Geometry check sheet. Reference: the model listing, model coordinates, mm. A direction names the side the tool comes from. Coordinates: 2 decimals unless noted, no trailing zeros. Loops run counter-clockwise (first coordinate to the right, second up) from the corner with the lowest first, then second, coordinate; pieces in that order, holes last.
from build123d import *

# Parameters (mm, degrees)
SKETCH1_W                     = 154
SKETCH1_H                     = 100
BOSS_EXTRUDE1_DEPTH           = 4
SKETCH2_R                     = 1.65
CUT_EXTRUDE1_DEPTH            = 184.66273438
SKETCH3_R                     = 7.5
BOSS_EXTRUDE2_DEPTH           = 6
BOSS_EXTRUDE2_DRAFT           = 15
BOSS_EXTRUDE2_PROFILE_2_DEPTH = 6
BOSS_EXTRUDE2_PROFILE_2_DRAFT = 15
BOSS_EXTRUDE2_PROFILE_3_DEPTH = 6
BOSS_EXTRUDE2_PROFILE_3_DRAFT = 15
BOSS_EXTRUDE2_PROFILE_4_DEPTH = 6
BOSS_EXTRUDE2_PROFILE_4_DRAFT = 15
SKETCH4_R                     = 3
CUT_EXTRUDE2_DEPTH            = 1.5


with BuildPart() as part:
    # Sketch1 → Boss-Extrude1 (new body)
    with BuildSketch(Plane(origin=(0, 0, 0), x_dir=(0, 1, 0), z_dir=(0, 0, 1))):
        with Locations((77, 50)):
            Rectangle(SKETCH1_W, SKETCH1_H)
    extrude(amount=BOSS_EXTRUDE1_DEPTH)

    # Sketch2 → Cut-Extrude1 (cut, through all)
    with BuildSketch(Plane(origin=(0, 0, 0), x_dir=(1, 0, 0), z_dir=(0, 0, -1))):
        with Locations(Location((-4, -77, 0), (0, 0, 180))):
            Circle(SKETCH2_R)
        with Locations(Location((-4, -17, 0), (0, 0, 180))):
            Circle(SKETCH2_R)
        with Locations(Location((-4, -137, 0), (0, 0, 180))):
            Circle(SKETCH2_R)
        with Locations(Location((-96, -137, 0), (0, 0, 180))):
            Circle(SKETCH2_R)
        with Locations(Location((-96, -77, 0), (0, 0, 180))):
            Circle(SKETCH2_R)
        with Locations(Location((-96, -17, 0), (0, 0, 180))):
            Circle(SKETCH2_R)
        with Locations(Location((-52, -97, 0), (0, 0, 180))):
            Circle(SKETCH2_R)
        with Locations(Location((-52, -57, 0), (0, 0, 180))):
            Circle(SKETCH2_R)
    extrude(amount=-CUT_EXTRUDE1_DEPTH, mode=Mode.SUBTRACT)


with BuildPart() as boss_extrude2_tool:
    # Sketch3 → Boss-Extrude2 (with draft: the straight prism first)
    with BuildSketch(Plane(origin=(0, 0, 0), x_dir=(1, 0, 0), z_dir=(0, 0, -1))):
        with Locations((-85, -15)):
            Circle(SKETCH3_R)
    extrude(amount=BOSS_EXTRUDE2_DEPTH)
    # Boss-Extrude2: the draft: its side faces are tilted about the plane it starts from
    boss_extrude2_sides = [boss_extrude2_tool.faces().sort_by_distance(p)[0] for p in [
        (-92.5, 15, -3),
    ]]
    draft(boss_extrude2_sides, Plane(origin=(0, 0, 0), x_dir=(1, 0, 0), z_dir=(0, 0, -1)), BOSS_EXTRUDE2_DRAFT)


with BuildPart() as part_1:
    add(part.part)

    # Boss-Extrude2: add boss_extrude2_tool
    add(boss_extrude2_tool.part)


with BuildPart() as boss_extrude2_profile_2_tool:
    # Sketch3 → Boss-Extrude2 profile 2 (with draft: the straight prism first)
    with BuildSketch(Plane(origin=(0, 0, 0), x_dir=(1, 0, 0), z_dir=(0, 0, -1))):
        with Locations((-15, -15)):
            Circle(SKETCH3_R)
    extrude(amount=BOSS_EXTRUDE2_PROFILE_2_DEPTH)
    # Boss-Extrude2 profile 2: the draft: its side faces are tilted about the plane it starts from
    boss_extrude2_profile_2_sides = [boss_extrude2_profile_2_tool.faces().sort_by_distance(p)[0] for p in [
        (-22.5, 15, -3),
    ]]
    draft(boss_extrude2_profile_2_sides, Plane(origin=(0, 0, 0), x_dir=(1, 0, 0), z_dir=(0, 0, -1)), BOSS_EXTRUDE2_PROFILE_2_DRAFT)


with BuildPart() as part_2:
    add(part_1.part)

    # Boss-Extrude2 profile 2: add boss_extrude2_profile_2_tool
    add(boss_extrude2_profile_2_tool.part)


with BuildPart() as boss_extrude2_profile_3_tool:
    # Sketch3 → Boss-Extrude2 profile 3 (with draft: the straight prism first)
    with BuildSketch(Plane(origin=(0, 0, 0), x_dir=(1, 0, 0), z_dir=(0, 0, -1))):
        with Locations((-15, -139)):
            Circle(SKETCH3_R)
    extrude(amount=BOSS_EXTRUDE2_PROFILE_3_DEPTH)
    # Boss-Extrude2 profile 3: the draft: its side faces are tilted about the plane it starts from
    boss_extrude2_profile_3_sides = [boss_extrude2_profile_3_tool.faces().sort_by_distance(p)[0] for p in [
        (-22.5, 139, -3),
    ]]
    draft(boss_extrude2_profile_3_sides, Plane(origin=(0, 0, 0), x_dir=(1, 0, 0), z_dir=(0, 0, -1)), BOSS_EXTRUDE2_PROFILE_3_DRAFT)


with BuildPart() as part_3:
    add(part_2.part)

    # Boss-Extrude2 profile 3: add boss_extrude2_profile_3_tool
    add(boss_extrude2_profile_3_tool.part)


with BuildPart() as boss_extrude2_profile_4_tool:
    # Sketch3 → Boss-Extrude2 profile 4 (with draft: the straight prism first)
    with BuildSketch(Plane(origin=(0, 0, 0), x_dir=(1, 0, 0), z_dir=(0, 0, -1))):
        with Locations((-85, -139)):
            Circle(SKETCH3_R)
    extrude(amount=BOSS_EXTRUDE2_PROFILE_4_DEPTH)
    # Boss-Extrude2 profile 4: the draft: its side faces are tilted about the plane it starts from
    boss_extrude2_profile_4_sides = [boss_extrude2_profile_4_tool.faces().sort_by_distance(p)[0] for p in [
        (-92.5, 139, -3),
    ]]
    draft(boss_extrude2_profile_4_sides, Plane(origin=(0, 0, 0), x_dir=(1, 0, 0), z_dir=(0, 0, -1)), BOSS_EXTRUDE2_PROFILE_4_DRAFT)


with BuildPart() as part_4:
    add(part_3.part)

    # Boss-Extrude2 profile 4: add boss_extrude2_profile_4_tool
    add(boss_extrude2_profile_4_tool.part)

    # Sketch4 → Cut-Extrude2 (cut)
    with BuildSketch(Plane(origin=(0, 0, 0), x_dir=(1, 0, 0), z_dir=(0, 0, -1))):
        with Locations(Location((-96, -17, 0), (0, 0, 180))):
            Circle(SKETCH4_R)
        with Locations(Location((-4, -17, 0), (0, 0, 180))):
            Circle(SKETCH4_R)
        with Locations(Location((-4, -77, 0), (0, 0, 180))):
            Circle(SKETCH4_R)
        with Locations(Location((-96, -77, 0), (0, 0, 180))):
            Circle(SKETCH4_R)
        with Locations(Location((-96, -137, 0), (0, 0, 180))):
            Circle(SKETCH4_R)
        with Locations(Location((-4, -137, 0), (0, 0, 180))):
            Circle(SKETCH4_R)
        with Locations(Location((-52, -57, 0), (0, 0, 180))):
            Circle(SKETCH4_R)
        with Locations(Location((-52, -97, 0), (0, 0, 180))):
            Circle(SKETCH4_R)
    extrude(amount=-CUT_EXTRUDE2_DEPTH, mode=Mode.SUBTRACT)


solid = part_4.part
1) Access from +Z, -Z, +X, -X, +Y, -Y to the whole of each face (thin tool, end or side, straight path). Record for faces 1 (the flat face through (-53.3, 95.7, 1.5)), 2 (the cylindrical face through (-2.784, 18.115, 2.732)).
Data:
face 1: -Z
face 2: +Z, -Z
2) Material ranges on probe 1 along X at (y, z) = (137, 2.3); probe 2 along Z at (x, y) = (-10.5, 93); probe 3 along Y at (x, z) = (-82, -3.75), recorded low to high.
Data:
probe 1: x = -100 to -97.65, -94.35 to -5.65, -2.35 to 0
probe 2: z = 0 to 4
probe 3: y = 9.24 to 20.76, 133.24 to 144.76
3) Section check D-D on z = -3.25. Record the cut outline in (x, y), and give its area (3 significant figures).
Data:
outline: circle Ø13.26 at (-85, 15); circle Ø13.26 at (-85, 139); circle Ø13.26 at (-15, 15); circle Ø13.26 at (-15, 139)
area: 552 mm2
4) Depth check by flat-ended pin: pin 1 (1 mm diameter, centred on x = -25.5, y = 17, fed in from -Z); pin 2 (4 mm diameter, centred on x = -96, y = 137, fed in from -Z); pin 3 (2 mm diameter, centred on x = -82, z = -3, fed in from -Y). Enter the tip coordinate at first touch or a pass-through.
Data:
pin 1: stops at z = 0
pin 2: stops at z = 1.5
pin 3: stops at y = 8.51
5) Section check C-C on y = 57. Record the cut outline in (x, z), and give its area (3 significant figures).
Data:
outline: (-100, 0) - (-55, 0) - (-55, 1.5) - (-53.65, 1.5) - (-53.65, 4) - (-100, 4) - close; (-50.35, 1.5) - (-49, 1.5) - (-49, 0) - (0, 0) - (0, 4) - (-50.35, 4) - close
area: 383 mm2
6) Section check A-A on y = 77. Record the cut outline in (x, z).
Data:
outline: (-100, 0) - (-99, 0) - (-99, 1.5) - (-97.65, 1.5) - (-97.65, 4) - (-100, 4) - close; (-94.35, 1.5) - (-93, 1.5) - (-93, 0) - (-7, 0) - (-7, 1.5) - (-5.65, 1.5) - (-5.65, 4) - (-94.35, 4) - close; (-2.35, 1.5) - (-1, 1.5) - (-1, 0) - (0, 0) - (0, 4) - (-2.35, 4) - close
7) Mould release check, pull along X, two halves, no side actions. Record for faces 3 (the cylindrical face through (-4.761, 135.536, 2.732)), 4 (the flat face through (-15, 15, -6)): +X half, -X half, draft (parallel to the pull), parting line (faces both ways), or undercut.
Data:
face 3: undercut
face 4: draft
8) Section check B-B on x = -96. Record the cut outline in (y, z).
Data:
outline: (0, 0) - (14, 0) - (14, 1.5) - (15.35, 1.5) - (15.35, 4) - (0, 4) - close; (18.65, 1.5) - (20, 1.5) - (20, 0) - (74, 0) - (74, 1.5) - (75.35, 1.5) - (75.35, 4) - (18.65, 4) - close; (78.65, 1.5) - (80, 1.5) - (80, 0) - (134, 0) - (134, 1.5) - (135.35, 1.5) - (135.35, 4) - (78.65, 4) - close; (138.65, 1.5) - (140, 1.5) - (140, 0) - (154, 0) - (154, 4) - (138.65, 4) - close
